Input: part model. Units: mm. Frame: model coordinates. Face numbers are marked on the shaded views. A direction names the side the tool comes from. Round coordinates to 2 decimals unless told otherwise and drop trailing zeros. Loops run counter-clockwise (first coordinate to the right, second up) from the corner with the lowest first, then second, coordinate; pieces in that order, holes last. Notation, with made-up numbers: M -1,73.5 L 54,73.5 A21 ccw 54,89.5 Z; hole C 63,24.25 d9. An arc over 180 degrees is marked long. Use one line per item in the form item = value. Start each with the question number.
Q1. Section query D-D, the plane z = 21.5. Output: boundary loops of the cut face in (x, y).
Q2. Section query B-B, the plane z = 2.75. Output: boundary loops of the cut face in (x, y) (1 decimal).
Q3. Section query A-A, the plane y = 6. Output: boundary loops of the cut face in (x, z) (3 decimals).
Q4. First-contact query: P1, Ø6, axis at x = 3, z = 14.5, coming from the -Y side; P2, Ø1.5, axis at x = -1, y = 3.5, coming from the +Z side; P3, Ø1.5, axis at x = -1.5, y = -1, coming from the +Z side. Flat tips, straight axial feed; report the tip coordinate or a pass-through.
Q5. Section query C-C, the plane x = 6.75. Output: boundary loops of the cut face in (y, z) (3 decimals), and give its area (3 significant figures).
Q6. Access query for the marked faces 1, 2 and 3. Directions: +Z, -Z, +X, -X, +Y, -Y. A direction counts if a zero-diameter tool reaches every point of the face in a straight line with its end or side. Return the directions, or none.
Q7. Ray query, line 1 along Z through (x, y) = (7, -6) (3 decimals); line 2 along Z through (x, y) = (2, -7.5); line 3 along X through (y, z) = (1.5, 21). Return the intervals inside material, ascending.
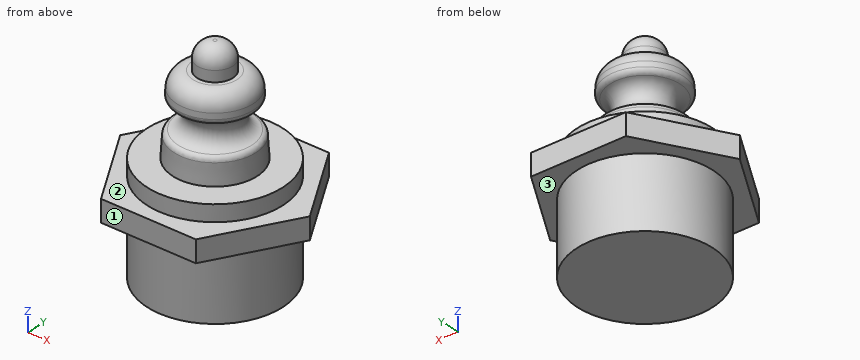
```python
from build123d import *

# Parameters (mm, degrees)
SKETCH1_R      = 7.9375
EXTRUDE1_DEPTH = 12.7
EXTRUDE2_DEPTH = 2.54
FILLET1_R      = 1.905
SKETCH5_R      = 2.092407527
EXTRUDE3_DEPTH = 3.175
FILLET2_R      = 1.905
FILLET3_R      = 0.635


with BuildPart() as part:
    # Sketch1 → Extrude1 (new body)
    with BuildSketch(Plane.XY):
        Circle(SKETCH1_R)
    extrude(amount=EXTRUDE1_DEPTH)

    # Sketch2 → Extrude2 (add)
    with BuildSketch(Plane.XY.offset(10.795)):
        Polygon((5.499261314, 9.525), (-5.499261314, 9.525), (-10.998522628, 0), (-5.499261314, -9.525), (5.499261314, -9.525), (10.998522628, 0), align=None)
    extrude(amount=-EXTRUDE2_DEPTH)

    # Sketch4 → Revolve1 (revolve)
    with BuildSketch(Plane(origin=(0, 0, 0), x_dir=(1, 0, 0), z_dir=(0, 1, 0))):
        with BuildLine():
            Line((-4.931059874, -12.7), (-4.747984705, -15.684208349))
            ThreePointArc((-4.747984705, -15.684208349), (-2.982016662, -17.246023592), (-4.543831906, -19.011991635))
            Line((-4.543831906, -19.011991635), (-4.360756736, -21.996199983))
            Line((-4.360756736, -21.996199983), (0, -21.996199983))
            Line((0, -21.996199983), (0, -12.7))
            Line((0, -12.7), (-4.931059874, -12.7))
        make_face()
    revolve(axis=Axis((0, 0, 12.7), (0, 0, 1)))

    # Fillet1
    fillet1_edges = [part.edges().sort_by_distance(p)[0] for p in [
        (4.360756736, 0, 21.996199983),
    ]]
    fillet(fillet1_edges, radius=FILLET1_R)

    # Sketch5 → Extrude3 (add)
    with BuildSketch(Plane.XY.offset(21.996199983)):
        Circle(SKETCH5_R)
    extrude(amount=EXTRUDE3_DEPTH)

    # Fillet2
    fillet2_edges = [part.edges().sort_by_distance(p)[0] for p in [
        (-2.092407527, 0, 25.171199983),
    ]]
    fillet(fillet2_edges, radius=FILLET2_R)

    # Fillet3
    fillet3_edges = [part.edges().sort_by_distance(p)[0] for p in [
        (4.747984705, 0, 15.684208349),
        (4.543831906, 0, 19.011991635),
    ]]
    fillet(fillet3_edges, radius=FILLET3_R)


solid = part.part
```
Results found:
q1.outline = C 0,0 d7.7
q2.outline = C 0,0 d15.9
q3.outline = M -7.534,8.255 L -5.197,8.255 L -5.197,0 L 5.197,0 L 5.197,8.255 L 7.534,8.255 L 7.534,10.795 L 5.197,10.795 L 5.197,12.7 L -5.197,12.7 L -5.197,10.795 L -7.534,10.795 Z
q4.P1 = -7.91
q4.P2 = 21.97
q4.P3 = 24.96
q5.outline = M -7.359,8.255 L -4.176,8.255 L -4.176,0 L 4.176,0 L 4.176,8.255 L 7.359,8.255 L 7.359,10.795 L 4.176,10.795 L 4.176,12.7 L -4.176,12.7 L -4.176,10.795 L -7.359,10.795 Z
q5.area = 122 mm²
q6.face_1 = +Z, -Z, +X, -X, -Y
q6.face_2 = +Z
q6.face_3 = -Z
q7.line_1 = 8.255 to 10.795
q7.line_2 = 0 to 12.7
q7.line_3 = -3.97 to 3.97
